The listing builds one solid part. Answer for the finished solid, in the listing's coordinates (mm). Face numbers are marked on the shaded views. A direction names the side the tool comes from. Give positions to 0.01 mm unless a question says otherwise; leave off trailing zeros. Write each loop counter-clockwise with the first axis right and the second up, starting at its lowest first coordinate (ties: lowest second). Pieces come first, ordered by that corner, then holes. Notation, with made-up numbers: (-30.75, 24) -> (14.25, 24) arc R30 ccw to (14.25, 56) -> close; hole circle Ø5 at (41, -38). An arc over 180 degrees is marked (long way). Put each result on its own line as item: value. Start each with the question number.
1) A flat-ended cylindrical pin translates along its axis: pin 1 Ø2 at (x, z) = (9.5, 18) entering from +Y. Find the tip coordinate at first contact, or state that the pin passes through.
2) A cutting plane is placed at A-A (z = 9). Write down the section's boundary in (x, y), then the cut area to 3 significant figures.
3) For the marked faces 1 and 2, determine the directions among +Z, -Z, +X, -X, +Y, -Y from which every point of the face is accessible in a straight line to the end or side of a thin tool.
4) A cutting plane is placed at B-B (x = 13.5). Write down the section's boundary in (y, z), then the cut area to 3 significant figures.
5) A cutting plane is placed at C-C (y = -1). Write down the section's boundary in (x, z) (3 decimals), then the cut area to 3 significant figures.
6) Find the intervals of material crossed by line 1 along Y through (x, z) = (13.5, 15.75); line 2 along X through (y, z) = (24.5, 11.75); line 3 along X through (y, z) = (5, 7.25) (3 decimals), in increasing order. Write a range as from..to.
7) A cutting plane is placed at D-D (z = 2). Write down the section's boundary in (x, y), then the cut area to 3 significant figures.
from build123d import *

# Parameters (mm, degrees)
F1_DEPTH = 25
F2_R     = 5
F3_R     = 5


with BuildPart() as f1:
    # F0 (on Top) → F1 (new body)
    with BuildSketch(Plane.XY):
        Polygon((-24.206446, 26.655727), (-34.206446, 26.655727), (-34.206446, -13.344273), (25.793554, -13.344273), (25.793554, -3.344273), (-4.206446, -3.344273), (-24.206446, 6.655727), align=None)
    extrude(amount=F1_DEPTH)

    # F2
    f2_edges = [f1.edges().sort_by_distance(p)[0] for p in [
        (-29.206446, 26.655727, 25),
        (-29.206446, 26.655727, 0),
    ]]
    fillet(f2_edges, radius=F2_R)

    # F3
    f3_edges = [f1.edges().sort_by_distance(p)[0] for p in [
        (25.793554, -8.344273, 25),
        (25.793554, -8.344273, 0),
    ]]
    fillet(f3_edges, radius=F3_R)


solid = f1.part
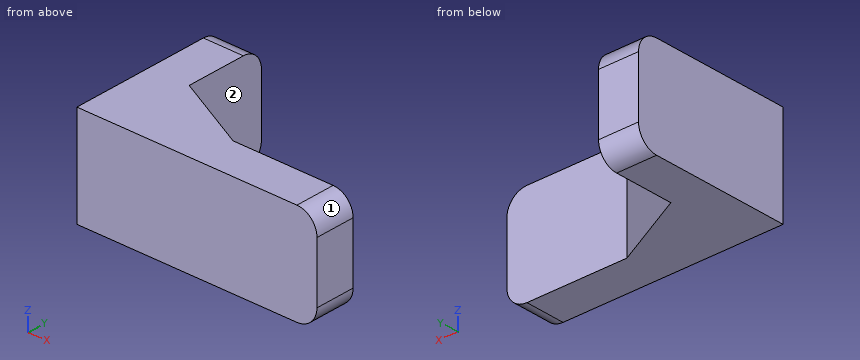
Reply:
1. pin 1: stops at y = -3.34
2. outline: (-34.21, -13.34) -> (25.79, -13.34) -> (25.79, -3.34) -> (-4.21, -3.34) -> (-24.21, 6.66) -> (-24.21, 26.66) -> (-34.21, 26.66) -> close
2. area: 1,000 mm2
3. face 1: +Z, +X, +Y, -Y
3. face 2: +Z, -Z, +X, +Y
4. outline: (-13.34, 0) -> (-3.34, 0) -> (-3.34, 25) -> (-13.34, 25) -> close
4. area: 250 mm2
5. outline: (-34.206, 0) -> (-8.895, 0) -> (-8.895, 25) -> (-34.206, 25) -> close
5. area: 633 mm2
6. line 1: y = -13.34..-3.34
6. line 2: x = -34.21..-24.21
6. line 3: x = -34.206..-20.895
7. outline: (-34.21, -13.34) -> (24.79, -13.34) -> (24.79, -3.34) -> (-4.21, -3.34) -> (-24.21, 6.66) -> (-24.21, 25.66) -> (-34.21, 25.66) -> close
7. area: 980 mm2
